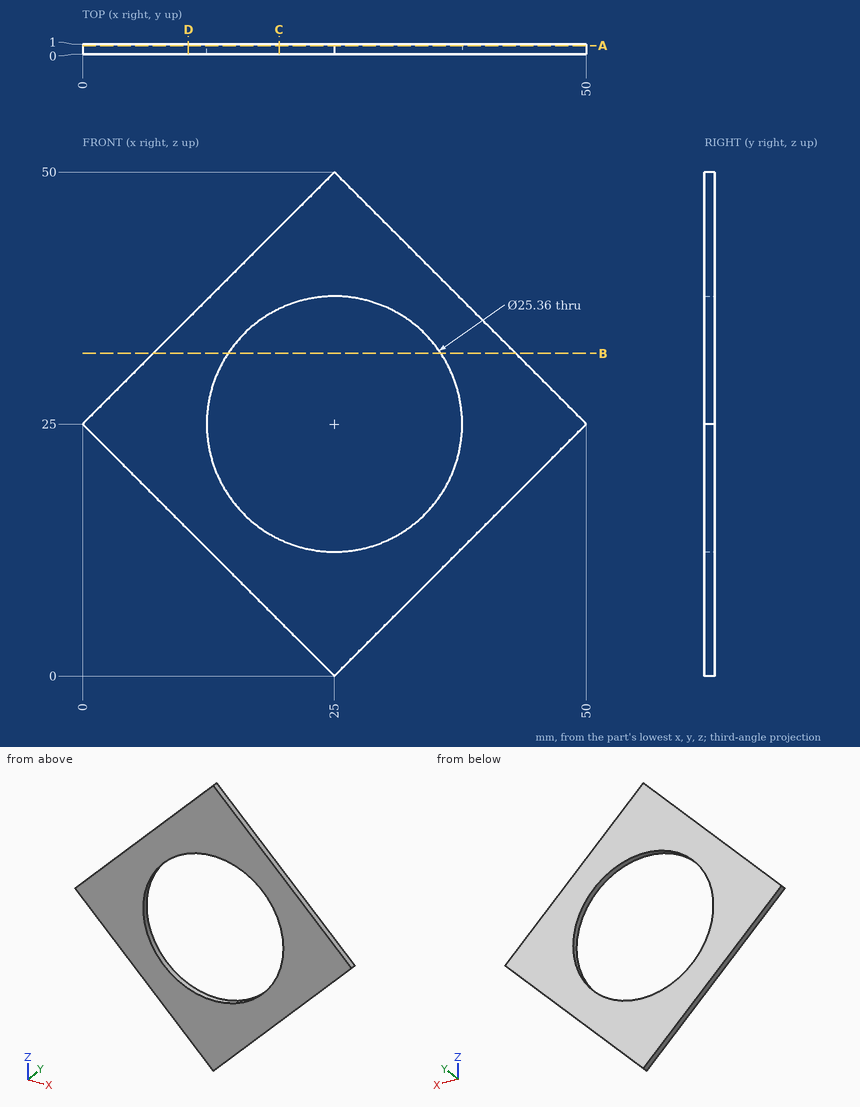
The drawing under review shows one solid part. Ordinate dimensions are in mm from its lowest x, y, z. Give positions to 0.01 mm unless a question says otherwise; leave off trailing zeros. Write each loop counter-clockwise with the first axis right and the second up, starting at its lowest first coordinate (ties: lowest second). Pieces come first, ordered by that corner, then holes.
1. For P1, Ø15, axis at x = 25, z = 25, coming from the -Y side, flat-tipped, find the tip position at first contact; note if it passes through.
2. Add section B-B, the plane z = 32. Write out the cut boundary in (x, y), plus the area to 3 significant figures.
3. Add section D-D, the plane x = 10.5. Write out the cut boundary in (y, z), plus the area to 3 significant figures.
4. Wall thickness on L1, parallel to X at y = 0.05, z = 31; L2, parallel to Z at x = 26, y = 0.2; L3, parallel to X at y = 0.9, z = 34: over which ranges is each line inside the solid? List them lowest first.
5. Add section A-A, the plane y = 0.85. Write out the cut boundary in (x, z).
6. Add section C-C, the plane x = 19.5. Write out the cut boundary in (y, z) (3 decimals), plus the area to 4 significant figures.
Worked answers:
1. P1: passes through
2. outline: (7, 0) - (14.43, 0) - (14.43, 1) - (7, 1) - close; (35.57, 0) - (43, 0) - (43, 1) - (35.57, 1) - close
2. area: 14.9 mm2
3. outline: (0, 14.5) - (1, 14.5) - (1, 35.5) - (0, 35.5) - close
3. area: 21.0 mm2
4. L1: x = 6 to 13.83, 36.17 to 44
4. L2: z = 1 to 12.36, 37.64 to 49
4. L3: x = 9 to 16.07, 33.93 to 41
5. outline: (0, 25) - (25, 0) - (50, 25) - (25, 50) - close; hole circle Ø25.36 at (25, 25)
6. outline: (0, 5.5) - (1, 5.5) - (1, 13.575) - (0, 13.575) - close; (0, 36.425) - (1, 36.425) - (1, 44.5) - (0, 44.5) - close
6. area: 16.15 mm2
